```python
from build123d import *

# Parameters (mm, degrees)
SKETCH_1_W             = 120
SKETCH_1_H             = 60
EXTRUDE_1_DEPTH        = 2
SKETCH_2_W             = 8
SKETCH_2_H             = 60
EXTRUDE_2_DEPTH        = 6
HOLE_WIZARD_M3_1_D     = 2.5
HOLE_WIZARD_M3_1_DEPTH = 8.5
HOLE_WIZARD_M3_1_TIP   = 0.751075774
HOLE_WIZARD_M4_1_D     = 3.3


with BuildPart() as part:
    # 草图1 → 凸台-拉伸1 (new body)
    with BuildSketch(Plane(origin=(0, 0, 0), x_dir=(1, 0, 0), z_dir=(0, 1, 0))):
        Rectangle(SKETCH_1_W, SKETCH_1_H)
    extrude(amount=EXTRUDE_1_DEPTH)

    # 草图2 → 凸台-拉伸2 (add)
    with BuildSketch(Plane.XZ):
        with Locations((-36.5, 0)):
            Rectangle(SKETCH_2_W, SKETCH_2_H)
        with Locations((36.5, 0)):
            Rectangle(SKETCH_2_W, SKETCH_2_H)
    extrude(amount=EXTRUDE_2_DEPTH)

    # M3 螺纹孔1
    with Locations(Plane(origin=(0, -6, 0), x_dir=(-1, 0, 0), z_dir=(0, -1, 0))):
        with Locations((36.5, 5), (-36.5, 5)):
            Hole(HOLE_WIZARD_M3_1_D / 2, depth=HOLE_WIZARD_M3_1_DEPTH)
            with Locations((0, 0, -(HOLE_WIZARD_M3_1_DEPTH + HOLE_WIZARD_M3_1_TIP / 2))):  # 118° drill point
                Cone(0, HOLE_WIZARD_M3_1_D / 2, HOLE_WIZARD_M3_1_TIP, mode=Mode.SUBTRACT)

    # M4 螺纹孔1 (through all)
    with Locations(Plane(origin=(0, 2, 0), x_dir=(1, 0, 0), z_dir=(0, 1, 0))):
        with Locations((54, 0), (-11, 0)):
            Hole(HOLE_WIZARD_M4_1_D / 2)


solid = part.part
```
Here's how the part is built. I have some questions about the finished solid (model axes, mm). A direction names the side the tool comes from. Coordinates: 2 decimals unless noted, no trailing zeros. Order: outer loops, then holes, each group sorted by start corner. A loop starts at its lowest first (then second) coordinate and runs counter-clockwise, first axis right, second up.
1) Imagine slicing it at B-B on x = 54. List the corners of the cut face in (y, z) for me.
2) Imagine slicing it at C-C on z = -5. List the corners of the cut face in (x, y) for me.
3) Will these pins go through, and if not, where does the flat tip stop? pin 1 (2 mm diameter, centred on x = 36.5, z = -5, fed in from -Y); pin 2 (4 mm diameter, centred on x = -36.5, z = -5, fed in from +Y); pin 3 (6 mm diameter, centred on x = -50, z = 5.5, fed in from -Y); pin 4 (1.5 mm diameter, centred on y = -3.5, z = 14, fed in from +X).
4) Imagine slicing it at A-A on y = -2.75. List the corners of the cut face in (x, z) for me, and give its area (3 significant figures).
5) Which directions (+Z, -Z, +X, -X, +Y, -Y) give clear straight access to the entire face, cutting with the end or side of a thin tool? Please do faces 1 (the face through (-1, 2, 0)), 2 (the face through (-40.5, -3, 0)), 3 (the face through (-12.524, 0.986, 0.632)), 4 (the face through (32.5, -3, 0)), 5 (the face through (50, 0, 0)).
6) We'd pull the mould along Z, two halves only. Please class faces 6 (the face through (40.5, -3, 0)), 7 (the face through (35.51, -1.94, -4.24)), 8 (the face through (55.65, 0.99, -0.07)), 9 (the face through (0, 1, 30)): +Z half, -Z half, draft (parallel to the pull), parting line (faces both ways), or undercut.
7) I need wall thicknesses on line 1 (X direction, y = 0.5, z = -5); line 2 (X direction, y = -1.75, z = -5); line 3 (X direction, y = -1.25, z = 12.5). Which ranges of each line are inside material? Lowest first, please.
8) Imagine slicing it at D-D on x = 36.5. List the corners of the cut face in (y, z) for me.
Response values:
1. outline: (0, -30) - (2, -30) - (2, -1.65) - (0, -1.65) - close; (0, 1.65) - (2, 1.65) - (2, 30) - (0, 30) - close
2. outline: (-60, 0) - (-40.5, 0) - (-40.5, -6) - (-37.75, -6) - (-37.75, 2) - (-60, 2) - close; (-35.25, -6) - (-32.5, -6) - (-32.5, 0) - (32.5, 0) - (32.5, -6) - (35.25, -6) - (35.25, 2) - (-35.25, 2) - close; (37.75, -6) - (40.5, -6) - (40.5, 0) - (60, 0) - (60, 2) - (37.75, 2) - close
3. pin 1: passes through
3. pin 2: stops at y = 2
3. pin 3: stops at y = 0
3. pin 4: stops at x = 40.5
4. outline: (-40.5, -30) - (-32.5, -30) - (-32.5, 30) - (-40.5, 30) - close; (32.5, -30) - (40.5, -30) - (40.5, 30) - (32.5, 30) - close; hole circle Ø2.5 at (-36.5, -5); hole circle Ø2.5 at (36.5, -5)
4. area: 950 mm2
5. face 1: +Z, -Z, +X, -X, +Y
5. face 2: +Z, -Z, -X, -Y
5. face 3: +Y, -Y
5. face 4: +Z, -Z, -Y
5. face 5: +Z, -Z, +X, -Y
6. face 6: draft
6. face 7: undercut
6. face 8: undercut
6. face 9: +Z half
7. line 1: x = -60 to -37.75, -35.25 to 35.25, 37.75 to 60
7. line 2: x = -40.5 to -37.75, -35.25 to -32.5, 32.5 to 35.25, 37.75 to 40.5
7. line 3: x = -40.5 to -32.5, 32.5 to 40.5
8. outline: (-6, -30) - (2, -30) - (2, -6.25) - (-6, -6.25) - close; (-6, -3.75) - (2, -3.75) - (2, 30) - (-6, 30) - close
